The model under review builds one solid part; all positions refer to its coordinate system, in mm. Face numbers are marked on the shaded views. Round coordinates to 2 decimals unless told otherwise and drop trailing zeros. Order: outer loops, then holes, each group sorted by start corner. A loop starts at its lowest first (then second) coordinate and runs counter-clockwise, first axis right, second up.
1) Consider section B-B (y = 15.5). Give the boundary of the cut face in (x, z).
2) Clearance check with flat-ended pins moving along their axes: P1, Ø2, axis at x = -6.5, y = -0.5, coming from the -Z side; P2, Ø1.8, axis at x = 15.5, y = -15.5, coming from the +Z side. State where each tip first meets the part, or that it passes through.
3) Consider section C-C (x = 15.5). Give the boundary of the cut face in (y, z).
4) Consider section D-D (z = 3.9). Give the boundary of the cut face in (x, y), then the cut area to 3 significant figures.
5) To check wall thickness, follow L1, parallel to Y at x = 15.5, z = 1.45; L2, parallel to Y at x = 0, z = 3.05; L3, parallel to Y at x = -14.5, z = 2.85. State the ranges of each line that lie inside material, in increasing order.
6) Mouldability with a two-part tool opening along Y and no side actions: class the marked faces 1, 2 and 3 as pulls with the +Y half, pulls with the -Y half, needs draft (parallel to the pull), parting line crosses it, or undercut.
7) Consider section A-A (x = 0). Give the boundary of the cut face in (y, z).
from build123d import *

# Parameters (mm, degrees)
F0_W     = 42.3
F0_H     = 51.15
F0_R     = 1.5
F0_R_2   = 5
F1_DEPTH = 6


with BuildPart() as f1:
    # F0 (on Top) → F1 (new body)
    with BuildSketch(Plane.XY):
        with Locations((0, -4.425)):
            Rectangle(F0_W, F0_H)
        with Locations((-15.5, -15.5)):
            Circle(F0_R, mode=Mode.SUBTRACT)
        with Locations((15.5, -15.5)):
            Circle(F0_R, mode=Mode.SUBTRACT)
        with Locations((-15.5, 15.5)):
            Circle(F0_R, mode=Mode.SUBTRACT)
        Circle(F0_R_2, mode=Mode.SUBTRACT)
        with Locations((15.5, 15.5)):
            Circle(F0_R, mode=Mode.SUBTRACT)
    extrude(amount=F1_DEPTH)


solid = f1.part
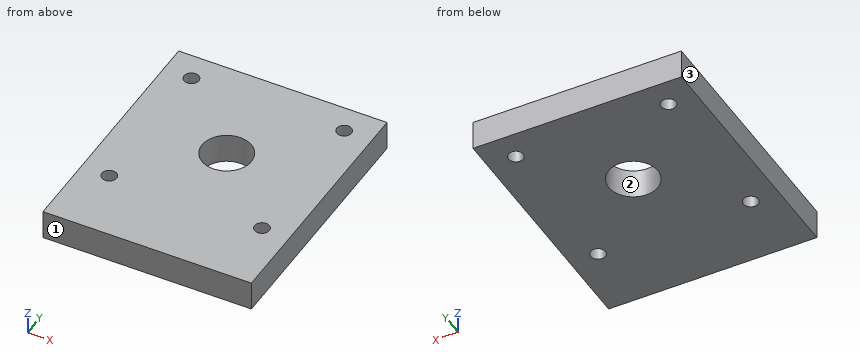
Answer below:
1. outline: (-21.15, 0) - (-17, 0) - (-17, 6) - (-21.15, 6) - close; (-14, 0) - (14, 0) - (14, 6) - (-14, 6) - close; (17, 0) - (21.15, 0) - (21.15, 6) - (17, 6) - close
2. P1: stops at z = 0
2. P2: passes through
3. outline: (-30, 0) - (-17, 0) - (-17, 6) - (-30, 6) - close; (-14, 0) - (14, 0) - (14, 6) - (-14, 6) - close; (17, 0) - (21.15, 0) - (21.15, 6) - (17, 6) - close
4. outline: (-21.15, -30) - (21.15, -30) - (21.15, 21.15) - (-21.15, 21.15) - close; hole circle Ø3 at (-15.5, -15.5); hole circle Ø3 at (-15.5, 15.5); hole circle Ø10 at (0, 0); hole circle Ø3 at (15.5, -15.5); hole circle Ø3 at (15.5, 15.5)
4. area: 2,060 mm2
5. L1: y = -30 to -17, -14 to 14, 17 to 21.15
5. L2: y = -30 to -5, 5 to 21.15
5. L3: y = -30 to -16.62, -14.38 to 14.38, 16.62 to 21.15
6. face 1: pulls with the -Y half
6. face 2: undercut
6. face 3: needs draft
7. outline: (-30, 0) - (-5, 0) - (-5, 6) - (-30, 6) - close; (5, 0) - (21.15, 0) - (21.15, 6) - (5, 6) - close
